Work out the finished part from the listing and answer in its coordinate system (mm). Coordinates: 2 decimals unless noted, no trailing zeros. Write each loop counter-clockwise with the first axis right and the second up, starting at its lowest first coordinate (ties: lowest second). Pieces come first, ordered by that corner, then holes. Notation, with made-up numbers: M 1.25,-32 L 16.25,-32 A25 ccw 16.25,-5 Z; hole C 73,-25.5 d3. An arc over 180 degrees is marked long. Answer as CSV lines item,"result". Start each with the question number.
(1) A cutting plane is placed at D-D on x = 125. Give the vertices of the cut face in (y, z), then the cut area to 3 significant figures.
(2) A cutting plane is placed at A-A on x = 162. Give the vertices of the cut face in (y, z).
(3) Flat-ended cylindrical pins translate along their axes: P1, Ø1.5, axis at x = 98, y = 2, coming from the +Z side; P2, Ø5, axis at x = 3, z = -92, coming from the -Y side; P3, Ø2, axis at x = 122.5, y = -22.5, coming from the +Z side; P4, Ø2.5, axis at x = 162, z = -3, coming from the -Y side. Find the tip coordinate at first contact, or state that the pin passes through.
(4) A cutting plane is placed at B-B on z = -92. Give the vertices of the cut face in (x, y).
(5) Find the intervals of material crossed by L1, parallel to X at y = 0.85, z = -3; L2, parallel to Z at x = 3, y = 1.15; L3, parallel to Y at x = 13, z = -89.5, in increasing order. Write a range as [from, to].
(6) A cutting plane is placed at C-C on z = -34.5. Give the vertices of the cut face in (x, y).
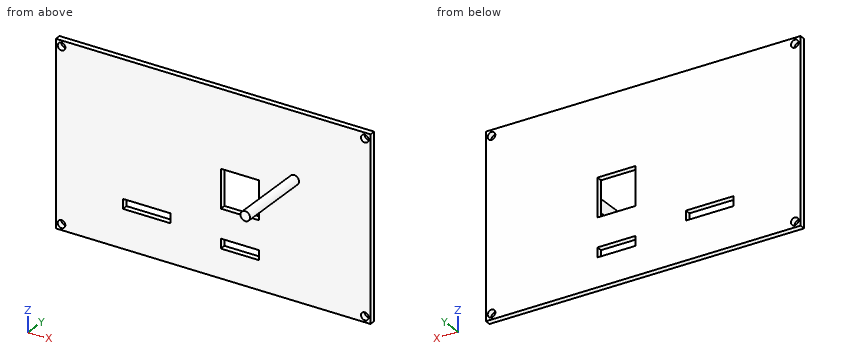
Autodesk Inventor part; units mm, degrees
ref_plane "YZ Plane" through (0, 0, 0) normal (1, 0, 0) x (0, 1, 0)
ref_plane "XZ Plane" through (0, 0, 0) normal (0, 1, 0) x (-1, 0, 0)
ref_plane "XY Plane" through (0, 0, 0) normal (0, 0, 1) x (1, 0, 0)
sketch "草圖1" plane through (0, 0, 0) normal (0, 1, 0) x (-1, 0, 0)
  line L0 (0, 0) -> (-165, 0)
  line L1 (-165, 0) -> (-165, -95)
  line L2 (-165, -95) -> (0, -95)
  line L3 (0, -95) -> (0, 0)
  dimension "d0" = 165
  dimension "d1" = 95
extrude "擠出1" add sketch "草圖1" along normal blind 3
sketch "草圖2" plane through (0, 3, 0) normal (0, 1, 0) x (1, 0, 0)
  line L0 (30, 75) -> (65, 75)
  line L1 (65, 75) -> (65, 20)
  line L2 (65, 20) -> (30, 20)
  line L3 (30, 20) -> (30, 75)
  line L4 (0, 95) -> (0, 0)
  line L5 (165, 95) -> (0, 95)
  line L6 (35.1505, 75) -> (60.1505, 75)
  line L7 (60.1505, 75) -> (60.1505, 70)
  line L8 (60.1505, 70) -> (35.1505, 70)
  line L9 (35.1505, 70) -> (35.1505, 75)
  dimension "d4" = 55
  dimension "d5" = 35
  dimension "d6" = 30
  dimension "d7" = 20
  dimension "d8" = 25
  dimension "d9" = 5
  dimension "d10" = 0
extrude "擠出2" cut sketch "草圖2" against normal blind 3 contours L0 L7 L8 L9
sketch "草圖3" plane through (0, 3, 0) normal (0, 1, 0) x (1, 0, 0)
  line L0 (86.5, 60) -> (106.5, 60)
  line L1 (106.5, 60) -> (106.5, 40)
  line L2 (106.5, 40) -> (86.5, 40)
  line L3 (86.5, 40) -> (86.5, 60)
  line L4 (85, 55) -> (108, 55)
  line L5 (108, 55) -> (108, 10)
  line L6 (108, 10) -> (85, 10)
  line L7 (85, 10) -> (85, 55)
  line L8 (165, 0) -> (165, 95)
  line L9 (0, 0) -> (165, 0)
  dimension "d13" = 20
  dimension "d14" = 20
  dimension "d15" = 23
  dimension "d16" = 45
  dimension "d17" = 80
  dimension "d18" = 1.5
  dimension "d19" = 30
  dimension "d20" = 10
extrude "擠出3" cut sketch "草圖3" against normal blind 3 contours L0 L1 L4 L3 | L4 L1 L2 L3
sketch "草圖4" plane through (0, 3, 0) normal (0, 1, 0) x (1, 0, 0)
  line L0 (86.5, 80) -> (106.5, 80)
  line L1 (106.5, 80) -> (106.5, 75)
  line L2 (106.5, 75) -> (86.5, 75)
  line L3 (86.5, 75) -> (86.5, 80)
  line L4 (86.5, 40) -> (86.5, 60)
  line L5 (106.5, 60) -> (106.5, 40)
  line L6 (86.5, 60) -> (106.5, 60)
  point P0 (0, 0)
  dimension "d23" = 0
  dimension "d24" = 0
  dimension "d25" = 5
  dimension "d26" = 15
extrude "擠出4" cut sketch "草圖4" against normal blind 3
sketch "草圖5" plane through (0, 3, 0) normal (0, 1, 0) x (1, 0, 0)
  circle A0 centre (3, 3) radius 2
  line L0 (0, 95) -> (0, 0)
  line L1 (0, 0) -> (165, 0)
  circle A1 centre (3, 92) radius 2
  line L2 (165, 95) -> (0, 95)
  circle A2 centre (162, 92) radius 2
  line L3 (165, 0) -> (165, 95)
  circle A3 centre (162, 3) radius 2
  dimension "d29" = 4
  dimension "d30" = 3
  dimension "d31" = 3
  dimension "d32" = 4
  dimension "d33" = 3
  dimension "d34" = 3
  dimension "d35" = 4
  dimension "d36" = 3
  dimension "d37" = 3
  dimension "d38" = 4
  dimension "d39" = 3
  dimension "d40" = 3
extrude "擠出5" cut sketch "草圖5" against normal blind 5 contours A0 | A1 | A2 | A3
sketch "草圖6" plane through (0, 0, 0) normal (0, -1, 0) x (1, 0, 0)
  circle A0 centre (125, -34.5) radius 2.5
  line L0 (165, 0) -> (165, -95)
  line L1 (0, 0) -> (165, 0)
  dimension "d43" = 5
  dimension "d44" = 40
  dimension "d45" = 32
extrude "擠出6" add sketch "草圖6" along normal blind 40
Here are the results:
1,outline,"M -40,-37 L 0,-37 L 0,-95 L 3,-95 L 3,0 L 0,0 L 0,-32 L -40,-32 Z"
1,area,"485 mm^2"
2,outline,"M 0,-95 L 3,-95 L 3,-94 L 0,-94 Z; M 0,-90 L 3,-90 L 3,-5 L 0,-5 Z; M 0,-1 L 3,-1 L 3,0 L 0,0 Z"
3,P1,"stops at z = 0"
3,P2,"stops at y = 0"
3,P3,"stops at z = -32.5"
3,P4,"passes through"
4,outline,"M 0,0 L 1,0 L 1,3 L 0,3 Z; M 5,0 L 160,0 L 160,3 L 5,3 Z; M 164,0 L 165,0 L 165,3 L 164,3 Z"
5,L1,"x = [0, 1], [5, 160], [164, 165]"
5,L2,"z = [-95, -94], [-90, -5], [-1, 0]"
5,L3,"y = [0, 3]"
6,outline,"M 0,0 L 122.5,0 L 122.5,-40 L 127.5,-40 L 127.5,0 L 165,0 L 165,3 L 0,3 Z"
